Here's how the part is built. I have some questions about the finished solid (model axes, mm). Face numbers are marked on the shaded views. Coordinates: 2 decimals unless noted, no trailing zeros. Loops run counter-clockwise (first coordinate to the right, second up) from the corner with the lowest first, then second, coordinate; pieces in that order, holes last. Notation, with made-up numbers: (73.5, 77) -> (119.5, 77) arc R16 cw to (119.5, 92) -> close; hole circle Ø8 at (5.5, 79). An arc over 180 degrees is marked (long way). Answer as a JSON object with one key per item and string values. Group by question number.
1) I want a section at A-A (z = 2). Count the separate pieces of the cut face and the enclosed holes in it, then the cut area to 3 significant figures.
2) I need wall thicknesses on probe 1 along X at (y, z) = (58.35, 8); probe 2 along Y at (x, z) = (34.5, 8.25); probe 3 along X at (y, z) = (43, 1.75). Which ranges of each line are inside material? Lowest first, please. Write a range as [from, to].
3) I want a section at C-C (x = 15.5). Write out the boundary of the cut face in (y, z), then the cut area to 3 significant figures.
4) I want a section at B-B (y = 27.35). Write out the boundary of the cut face in (x, z), then the cut area to 3 significant figures.
5) If we mould it in two halves opening along Y, with no side actions, what happens to the marked faces 1, 2 and 3? For each: +Y half, -Y half, draft (parallel to the pull), parting line (faces both ways), or undercut.
6) I want a section at D-D (y = 42.85). Write out the boundary of the cut face in (x, z), then the cut area to 3 significant figures.
7) I'm going to push flat-ended pins straight in: pin 1 (2 mm diameter, centred on x = 65.5, y = 27.35, fed in from +Z); pin 2 (11 mm diameter, centred on x = 46.5, y = 44, fed in from +Z); pin 3 (6 mm diameter, centred on x = 34.5, y = 27.35, fed in from +Z); pin 4 (3 mm diameter, centred on x = 65, y = 27, fed in from -Z). Where does each tip first touch, or does it pass through?
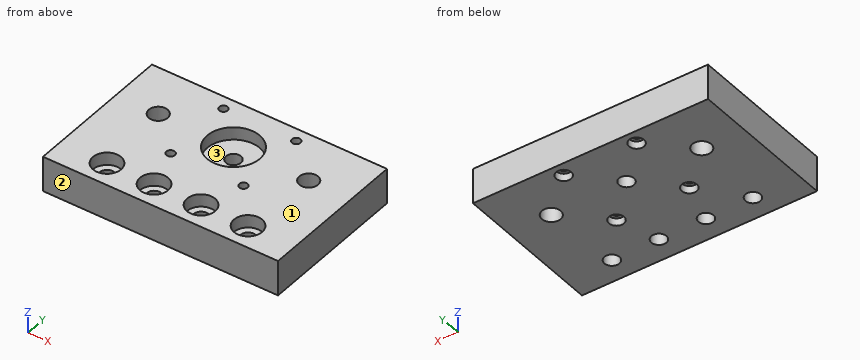
```python
from build123d import *

# Parameters (mm, degrees)
SKETCH_W        = 100
SKETCH_H        = 64
SKETCH_R        = 3.2
SKETCH_R_2      = 1.8
SKETCH_R_3      = 4
PAD_DEPTH       = 15
SKETCH001_R     = 11.2
SKETCH001_R_2   = 6
POCKET_DEPTH    = 5.4
SKETCH002_R     = 3.2
POCKET001_DEPTH = 3.2
SKETCH003_R     = 6
POCKET002_DEPTH = 5.4
SKETCH004_R     = 3.2
POCKET003_DEPTH = 15


with BuildPart() as part:
    # Sketch → Pad (new body)
    with BuildSketch(Plane.XY):
        with Locations((50, 32)):
            Rectangle(SKETCH_W, SKETCH_H)
        with Locations((50, 42.85)):
            Circle(SKETCH_R, mode=Mode.SUBTRACT)
        with Locations((65.5, 58.35)):
            Circle(SKETCH_R_2, mode=Mode.SUBTRACT)
        with Locations((65.5, 27.35)):
            Circle(SKETCH_R_2, mode=Mode.SUBTRACT)
        with Locations((34.5, 27.35)):
            Circle(SKETCH_R_2, mode=Mode.SUBTRACT)
        with Locations((34.5, 58.35)):
            Circle(SKETCH_R_2, mode=Mode.SUBTRACT)
        with Locations((20, 10)):
            Circle(SKETCH_R, mode=Mode.SUBTRACT)
        with Locations((80, 10)):
            Circle(SKETCH_R, mode=Mode.SUBTRACT)
        with Locations((82, 42.85)):
            Circle(SKETCH_R_3, mode=Mode.SUBTRACT)
        with Locations((18, 42.85)):
            Circle(SKETCH_R_3, mode=Mode.SUBTRACT)
    extrude(amount=PAD_DEPTH)

    # Sketch001 (on Face15 of Pad) → Pocket (cut)
    with BuildSketch(Plane.XY.offset(15)):
        with Locations((50, 42.85)):
            Circle(SKETCH001_R)
        with Locations((20, 10)):
            Circle(SKETCH001_R_2)
        with Locations((80, 10)):
            Circle(SKETCH001_R_2)
    extrude(amount=-POCKET_DEPTH, mode=Mode.SUBTRACT)

    # Sketch002 (on Face4 of Pocket) → Pocket001 (cut)
    with BuildSketch(Plane(origin=(0, 0, 0), x_dir=(1, 0, 0), z_dir=(0, 0, -1))):
        with Locations((34.5, -27.35)):
            Circle(SKETCH002_R)
        with Locations((65.5, -27.35)):
            Circle(SKETCH002_R)
        with Locations((34.5, -58.35)):
            Circle(SKETCH002_R)
        with Locations((65.5, -58.35)):
            Circle(SKETCH002_R)
    extrude(amount=-POCKET001_DEPTH, mode=Mode.SUBTRACT)

    # Sketch003 (on Face5 of Pocket001) → Pocket002 (cut)
    with BuildSketch(Plane.XY.offset(15)):
        with Locations((40, 10)):
            Circle(SKETCH003_R)
        with Locations((60, 10)):
            Circle(SKETCH003_R)
    extrude(amount=-POCKET002_DEPTH, mode=Mode.SUBTRACT)

    # Sketch004 (on Face4 of Pocket002) → Pocket003 (cut)
    with BuildSketch(Plane(origin=(0, 0, 0), x_dir=(1, 0, 0), z_dir=(0, 0, -1))):
        with Locations((40, -10)):
            Circle(SKETCH004_R)
        with Locations((60, -10)):
            Circle(SKETCH004_R)
    extrude(amount=-POCKET003_DEPTH, mode=Mode.SUBTRACT)


solid = part.part
```
Determined:
{
 "1": {"separate pieces": "1", "enclosed holes": "11", "area": "6,010 mm^2"},
 "2": {"probe 1": "[0, 32.7], [36.3, 63.7], [67.3, 100]", "probe 2": "[0, 25.55], [29.15, 56.55], [60.15, 64]", "probe 3": "[0, 14], [22, 46.8], [53.2, 78], [86, 100]"},
 "3": {"outline": "(0, 0) -> (39.73, 0) -> (39.73, 15) -> (13.97, 15) -> (13.97, 9.6) -> (6.03, 9.6) -> (6.03, 15) -> (0, 15) -> close; (45.97, 0) -> (64, 0) -> (64, 15) -> (45.97, 15) -> close", "area": "823 mm^2"},
 "4": {"outline": "(0, 0) -> (31.3, 0) -> (31.3, 3.2) -> (32.7, 3.2) -> (32.7, 15) -> (0, 15) -> close; (36.3, 3.2) -> (37.7, 3.2) -> (37.7, 0) -> (62.3, 0) -> (62.3, 3.2) -> (63.7, 3.2) -> (63.7, 15) -> (36.3, 15) -> close; (67.3, 3.2) -> (68.7, 3.2) -> (68.7, 0) -> (100, 0) -> (100, 15) -> (67.3, 15) -> close", "area": "1,370 mm^2"},
 "5": {"face 1": "draft", "face 2": "-Y half", "face 3": "undercut"},
 "6": {"outline": "(0, 0) -> (14, 0) -> (14, 15) -> (0, 15) -> close; (22, 0) -> (46.8, 0) -> (46.8, 9.6) -> (38.8, 9.6) -> (38.8, 15) -> (22, 15) -> close; (53.2, 0) -> (78, 0) -> (78, 15) -> (61.2, 15) -> (61.2, 9.6) -> (53.2, 9.6) -> close; (86, 0) -> (100, 0) -> (100, 15) -> (86, 15) -> close", "area": "1,080 mm^2"},
 "7": {"pin 1": "through", "pin 2": "z = 9.6", "pin 3": "z = 15", "pin 4": "z = 3.2"}
}
